Design review of the part built by this model. Coordinates are the model's own, in mm. Coordinates: 2 decimals unless noted, no trailing zeros. Order: outer loops, then holes, each group sorted by start corner. A loop starts at its lowest first (then second) coordinate and runs counter-clockwise, first axis right, second up. Notation, with made-up numbers: M 40.25,-27.75 L 97.25,-27.75 A31 ccw 97.25,7.25 Z; hole C 33,51.25 d3. An arc over 180 degrees is marked long. Answer as a JSON object with one key per item and string values.
from build123d import *

# Parameters (mm, degrees)
SKETCH2_R               = 25
BOSS_EXTRUDE1_DEPTH     = 12
CUT_EXTRUDE1_DEPTH      = 38.336309405
CUT_EXTRUDE1_DEPTH_BACK = 38.336309405
SKETCH3_R               = 3
CUT_EXTRUDE2_DEPTH      = 38.33630958
CUT_EXTRUDE2_DEPTH_BACK = 38.33630958
SKETCH4_R               = 16


with BuildPart() as part:
    # Sketch2 → Boss-Extrude1 (new body)
    with BuildSketch(Plane(origin=(0, 0, 0), x_dir=(1, 0, 0), z_dir=(0, 1, 0))):
        with Locations(Location((0, 0, 0), (0, 0, 270))):
            Circle(SKETCH2_R)
    extrude(amount=BOSS_EXTRUDE1_DEPTH)

    # Sketch3 → Cut-Extrude1 (cut, two sides: drawn at the far end of the back side and taken through both)
    with BuildSketch(Plane(origin=(0, 0, 0), x_dir=(0, 0, -1), z_dir=(1, 0, 0)).offset(-CUT_EXTRUDE1_DEPTH_BACK)):
        with Locations((0, 5.972869538)):
            Circle(SKETCH3_R)
    extrude(amount=CUT_EXTRUDE1_DEPTH + CUT_EXTRUDE1_DEPTH_BACK, mode=Mode.SUBTRACT)

    # Sketch4 → Cut-Extrude2 (cut, two sides: drawn at the far end of the back side and taken through both)
    with BuildSketch(Plane.XZ.offset(-CUT_EXTRUDE2_DEPTH_BACK)):
        with Locations(Location((0, 0, 0), (0, 0, 270))):
            Circle(SKETCH4_R)
    extrude(amount=CUT_EXTRUDE2_DEPTH + CUT_EXTRUDE2_DEPTH_BACK, mode=Mode.SUBTRACT)


solid = part.part
1) Insertion check: pin 1 Ø2 at (x, y) = (9, 3.5) entering from +Z; pin 2 Ø2 at (y, z) = (8.5, -13) entering from +X; pin 3 Ø5 at (x, y) = (-6, 6) entering from +Z. Each pin has a flat end and moves straight along its axis. Give the tip position at first contact, or say it passes through.
Taken from the geometry:
{"pin 1": "stops at z = 23.69", "pin 2": "stops at x = 21.93", "pin 3": "stops at z = 24.75"}
2) Add section A-A (x = 0). State the section outline as (y, z) points.
Taken from the geometry:
{"outline": "M 0,-25 L 12,-25 L 12,-16 L 0,-16 Z; M 0,16 L 12,16 L 12,25 L 0,25 Z"}
3) To check wall thickness, follow L1, parallel to Y at x = 23, z = 0; L2, parallel to Z at x = 9, y = 5.25; L3, parallel to Z at x = 17, y = 4.75. State the ranges of each line that lie inside material, in increasing order.
Taken from the geometry:
{"L1": "y = 0 to 2.97, 8.97 to 12", "L2": "z = -23.32 to -13.23, 13.23 to 23.32", "L3": "z = -18.33 to -2.74, 2.74 to 18.33"}
4) Mouldability with a two-part tool opening along Y and no side actions: class faces 1 (the cylindrical face through (20.295, 3.044, 0.65)), 2 (the flat face through (-16.3, 0, -0.4)), 3 (the flat face through (-16.3, 12, -0.4)) as released by +Y, released by -Y, zero draft, split by the parting line, or undercut.
Taken from the geometry:
{"face 1": "undercut", "face 2": "released by -Y", "face 3": "released by +Y"}
5) Add section B-B (z = 0). State the section outline as (x, y) points, and give its area (3 significant figures).
Taken from the geometry:
{"outline": "M -25,0 L -16,0 L -16,2.97 L -25,2.97 Z; M -25,8.97 L -16,8.97 L -16,12 L -25,12 Z; M 16,0 L 25,0 L 25,2.97 L 16,2.97 Z; M 16,8.97 L 25,8.97 L 25,12 L 16,12 Z", "area": "108 mm2"}
6) Add section D-D (y = 1). State the section outline as (x, z) points.
Taken from the geometry:
{"outline": "C 0,0 d50; hole C 0,0 d32"}
7) Add section C-C (y = 5.25). State the section outline as (x, z) points, and give its area (3 significant figures).
Taken from the geometry:
{"outline": "M -24.83,-2.91 A25 ccw 24.83,-2.91 L 15.73,-2.91 A16 cw -15.73,-2.91 Z; M -24.83,2.91 L -15.73,2.91 A16 cw 15.73,2.91 L 24.83,2.91 A25 ccw Z", "area": "1,050 mm2"}
